```python
from build123d import *

# Parameters (mm, degrees)
BOSS_EXTRUDE1_DEPTH = 3
SKETCH2_R           = 2.425
CUT_EXTRUDE1_DEPTH  = 3
BOSS_EXTRUDE3_DEPTH = 3
BOSS_EXTRUDE4_DEPTH = 2
SKETCH7_R           = 2.425
SKETCH7_R_2         = 2.2
CUT_EXTRUDE4_DEPTH  = 12


with BuildPart() as part:
    # Sketch1 → Boss-Extrude1 (new body)
    with BuildSketch(Plane.XY):
        with BuildLine():
            Line((3.15, 0), (24, 0))
            ThreePointArc((24, 0), (26.227386361, 0.922613639), (27.15, 3.15))
            Line((27.15, 3.15), (27.15, 34))
            Line((27.15, 34), (0, 34))
            Line((0, 34), (0, 3.15))
            ThreePointArc((0, 3.15), (0.922613639, 0.922613639), (3.15, 0))
        make_face()
    extrude(amount=BOSS_EXTRUDE1_DEPTH)

    # Sketch2 → Cut-Extrude1 (cut)
    with BuildSketch(Plane.XY.offset(3)):
        with Locations((5.575, 5.575)):
            Circle(SKETCH2_R)
        with Locations((13.575, 5.575)):
            Circle(SKETCH2_R)
        with Locations((21.575, 5.575)):
            Circle(SKETCH2_R)
        with Locations((13.575, 13.575)):
            Circle(SKETCH2_R)
        with Locations((21.575, 13.575)):
            Circle(SKETCH2_R)
        with Locations((5.575, 13.575)):
            Circle(SKETCH2_R)
        with Locations((13.575, 21.575)):
            Circle(SKETCH2_R)
        with Locations((21.575, 21.575)):
            Circle(SKETCH2_R)
        with Locations((5.575, 21.575)):
            Circle(SKETCH2_R)
        with Locations((5.575, 29.575)):
            Circle(SKETCH2_R)
        with Locations((13.575, 29.575)):
            Circle(SKETCH2_R)
        with Locations((21.575, 29.575)):
            Circle(SKETCH2_R)
    extrude(amount=-CUT_EXTRUDE1_DEPTH, mode=Mode.SUBTRACT)

    # Sketch3 → Boss-Extrude3 (add)
    with BuildSketch(Plane.XY):
        Polygon((0.024211768, 24.024211768), (9.71157467, 33.71157467), (-4.430560954, 47.853710294), (-14.117923856, 38.166347391), align=None)
        Polygon((17.43842533, 33.71157467), (26.524747468, 24.625252532), (40.666883092, 38.767388155), (31.580560954, 47.853710294), align=None)
    extrude(amount=BOSS_EXTRUDE3_DEPTH)

    # Sketch6 → Boss-Extrude4 (add)
    with BuildSketch(Plane.XY.offset(3)):
        Polygon((-14.117923856, 38.166347391), (0, 24.048423535), (0.707681609, 24.756105144), (-13.410242247, 38.874029), align=None)
        Polygon((-4.430560954, 47.853710294), (9.42314934, 34), (8.716042559, 33.292893219), (-5.137667735, 47.146603512), align=None)
        Polygon((17.72685066, 34), (31.580560954, 47.853710294), (32.287667735, 47.146603512), (18.433957441, 33.292893219), align=None)
        Polygon((27.15, 25.250505063), (40.666883092, 38.767388155), (39.959776311, 39.474494937), (26.442893219, 25.957611845), align=None)
    extrude(amount=BOSS_EXTRUDE4_DEPTH)

    # Sketch7 → Cut-Extrude4 (cut)
    with BuildSketch(Plane.XY.offset(3)):
        with Locations((5.575, 29.575)):
            Circle(SKETCH7_R)
        with Locations((21.575, 29.575)):
            Circle(SKETCH7_R)
        with Locations((-6.091687062, 39.828623155)):
            Circle(SKETCH7_R_2)
        with Locations((32.641221126, 40.429089091)):
            Circle(SKETCH7_R_2)
    extrude(amount=-CUT_EXTRUDE4_DEPTH, mode=Mode.SUBTRACT)


solid = part.part
```
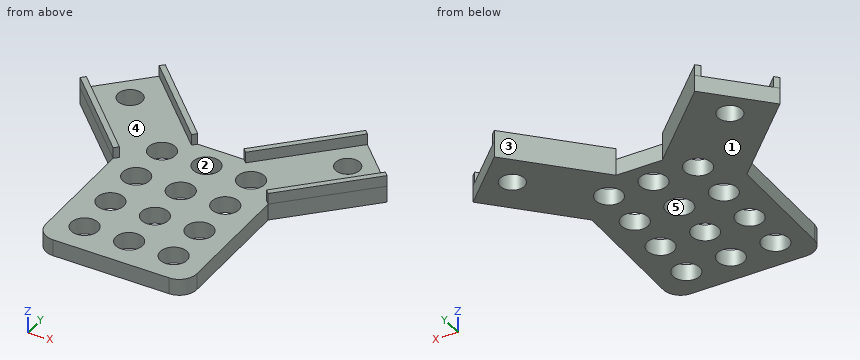
The listing builds one solid part. Answer for the finished solid, in the listing's coordinates (mm). Face numbers are marked on the shaded views. A direction names the side the tool comes from. Round coordinates to 2 decimals unless told otherwise and drop trailing zeros. Loops run counter-clockwise (first coordinate to the right, second up) from the corner with the lowest first, then second, coordinate; pieces in that order, holes last. Notation, with made-up numbers: (16, -7) - (60, -7) arc R10 cw to (60, 1) - close; hole circle Ø1 at (-30.75, 66.25). An arc over 180 degrees is marked (long way). Return JSON: item names as keys, results as strings. Group by question number.
1. The part is cut by section A-A on y = 30.5. Determine the outline of the cut face in (x, z), then the cut area to 3 significant figures.
2. Which of the six approach directions +Z, -Z, +X, -X, +Y, -Y give full straight-line access (tool end or side, diameter ignored) to the marked faces 4 and 5?
3. The mould has two halves that part along Y. Classify the marked faces 1, 2 and 3: pulls with the +Y half, pulls with the -Y half, needs draft (parallel to the pull), parting line crosses it, or undercut.
4. Each of these flat-tipped pins is pushed along its axis until it touches: P1, Ø3, axis at y = 31, z = 2.5, coming from the +X side; P2, Ø0.9, axis at y = 10, z = 1, coming from the -X side; P3, Ø5.5, axis at x = 13.575, y = 5.575, coming from the +Z side. Where does it stop, or does it pass through?
5. The part is cut by section C-C on z = 1.3. State how many separate pieces and enclosed holes the cut face has, then the cut area to 3 significant figures.
6. The part is cut by section B-B on x = 6.5. Determine the outline of the cut face in (y, z), then the cut area to 3 significant figures.
7. Consider probe 1 along X at (y, z) = (33.5, 4.35); probe 2 along Y at (x, z) = (5, 2.8); probe 3 along Y at (x, z) = (6, 0.9). Determine where each line is inside the solid, lowest interval first.
8. The part is cut by section D-D on x = 37.5. Determine the outline of the cut face in (y, z).
Resolved:
{
 "1": {"outline": "(-6.45, 0) - (3.33, 0) - (3.33, 3) - (-5.04, 3) - (-5.04, 5) - (-6.45, 5) - close; (7.82, 0) - (11.33, 0) - (11.33, 3) - (7.82, 3) - close; (15.82, 0) - (19.33, 0) - (19.33, 3) - (15.82, 3) - close; (23.82, 0) - (32.4, 0) - (32.4, 5) - (30.99, 5) - (30.99, 3) - (23.82, 3) - close", "area": "81.9 mm²"},
 "2": {"face 4": "+Z", "face 5": "+Z, -Z"},
 "3": {"face 1": "needs draft", "face 2": "undercut", "face 3": "pulls with the +Y half"},
 "4": {"P1": "stops at x = 34.4", "P2": "stops at x = 0", "P3": "stops at z = 3"},
 "5": {"separate pieces": "1", "enclosed holes": "14", "area": "1,100 mm²"},
 "6": {"outline": "(0, 0) - (3.33, 0) - (3.33, 3) - (0, 3) - close; (7.82, 0) - (11.33, 0) - (11.33, 3) - (7.82, 3) - close; (15.82, 0) - (19.33, 0) - (19.33, 3) - (15.82, 3) - close; (23.82, 0) - (27.33, 0) - (27.33, 3) - (23.82, 3) - close; (31.82, 0) - (36.92, 0) - (36.92, 5) - (35.51, 5) - (35.51, 3) - (31.82, 3) - close", "area": "59.8 mm²"},
 "7": {"probe 1": "x = -9.45 to -8.04, 8.51 to 8.92, 18.23 to 18.64, 33.99 to 35.4", "probe 2": "y = 0 to 3.22, 7.93 to 11.22, 15.93 to 19.22, 23.93 to 27.22, 31.93 to 38.42", "probe 3": "y = 0 to 3.19, 7.96 to 11.19, 15.96 to 19.19, 23.96 to 27.19, 31.96 to 37.42"},
 "8": {"outline": "(35.6, 0) - (41.93, 0) - (41.93, 3) - (37.01, 3) - (37.01, 5) - (35.6, 5) - close"}
}
